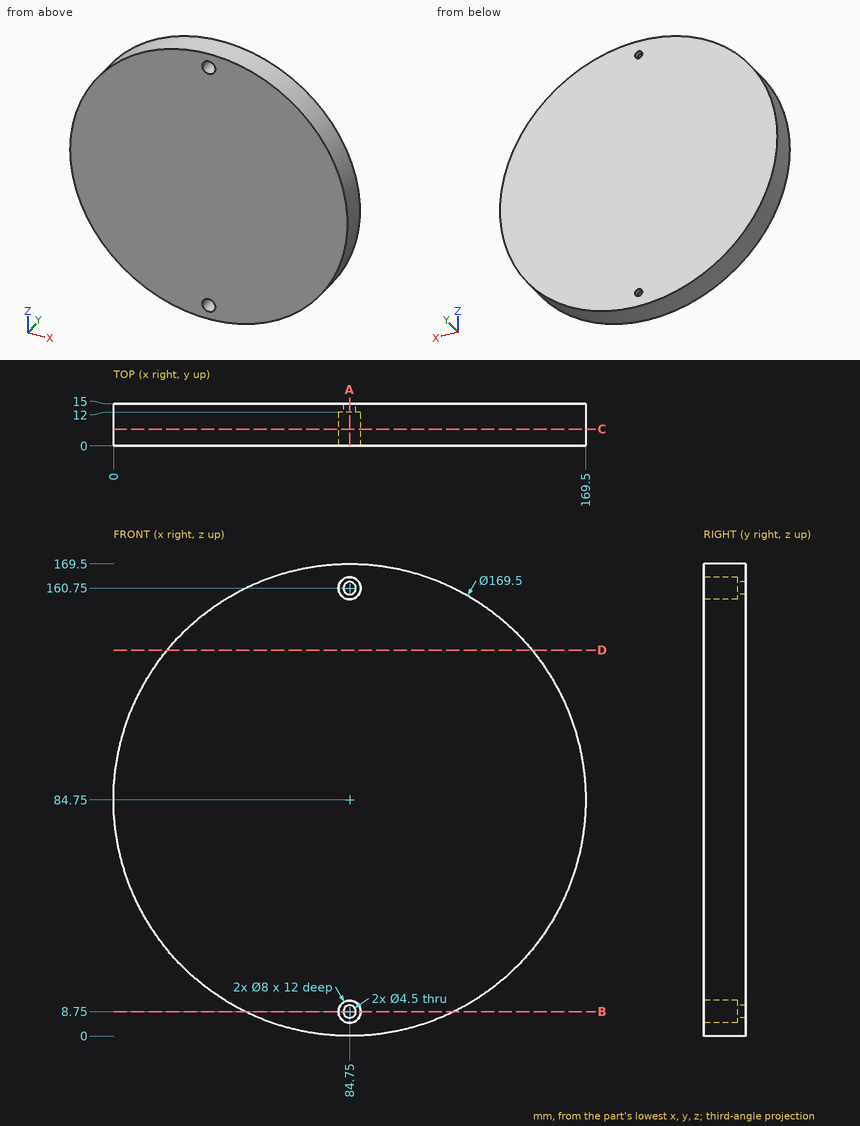
Here's the drawing with two shaded views (mm, measured from the low corner). I have some questions. Round coordinates to 2 decimals unless told otherwise and drop trailing zeros. Order: outer loops, then holes, each group sorted by start corner. A loop starts at its lowest first (then second) coordinate and runs counter-clockwise, first axis right, second up. Notation, with made-up numbers: (-38, 8) -> (-13, 8) arc R12 ccw to (-13, 29) -> close; hole circle Ø9 at (8.25, -17). An arc over 180 degrees is marked (long way). Write each question's results on one line, items separated by ' | '. Start each with the question number.
Item 1: If we section it at C-C, the plane y = 6: Write out the boundary of the cut face in (x, z).
Item 2: Will these pins go through, and if not, where does the flat tip stop? pin 1 (4 mm diameter, centred on x = 26.5, y = 7, fed in from +Z); pin 2 (3 mm diameter, centred on x = 99.5, y = 11.5, fed in from -Z); pin 3 (2.5 mm diameter, centred on x = 84.75, z = 160.75, fed in from +Y); pin 4 (3 mm diameter, centred on x = 77, y = 4, fed in from +Z).
Item 3: If we section it at B-B, the plane z = 8.75: Write out the boundary of the cut face in (x, y), then the cut area to 3 significant figures.
Item 4: Please list where these lines run through material, in increasing order: L1, parallel to Z at x = 84.75, y = 9; L2, parallel to Z at x = 84.75, y = 13.6; L3, parallel to X at y = 14.4, z = 160.75.
Item 5: If we section it at A-A, the plane x = 84.75: Write out the boundary of the cut face in (y, z), then the cut area to 3 significant figures.
Item 6: If we section it at D-D, the plane z = 138.5: Write out the boundary of the cut face in (x, y), then the cut area to 3 significant figures.
Results:
1) outline: circle Ø169.5 at (84.75, 84.75); hole circle Ø8 at (84.75, 8.75); hole circle Ø8 at (84.75, 160.75)
2) pin 1: stops at z = 148.14 | pin 2: stops at z = 1.04 | pin 3: passes through | pin 4: stops at z = 169.27
3) outline: (47.25, 0) -> (80.75, 0) -> (80.75, 12) -> (82.5, 12) -> (82.5, 15) -> (47.25, 15) -> close; (87, 12) -> (88.75, 12) -> (88.75, 0) -> (122.25, 0) -> (122.25, 15) -> (87, 15) -> close | area: 1,020 mm2
4) L1: z = 0 to 4.75, 12.75 to 156.75, 164.75 to 169.5 | L2: z = 0 to 6.5, 11 to 158.5, 163 to 169.5 | L3: x = 47.25 to 82.5, 87 to 122.25
5) outline: (0, 0) -> (15, 0) -> (15, 6.5) -> (12, 6.5) -> (12, 4.75) -> (0, 4.75) -> close; (0, 12.75) -> (12, 12.75) -> (12, 11) -> (15, 11) -> (15, 158.5) -> (12, 158.5) -> (12, 156.75) -> (0, 156.75) -> close; (0, 164.75) -> (12, 164.75) -> (12, 163) -> (15, 163) -> (15, 169.5) -> (0, 169.5) -> close | area: 2,320 mm2
6) outline: (19.23, 0) -> (150.27, 0) -> (150.27, 15) -> (19.23, 15) -> close | area: 1,970 mm2
